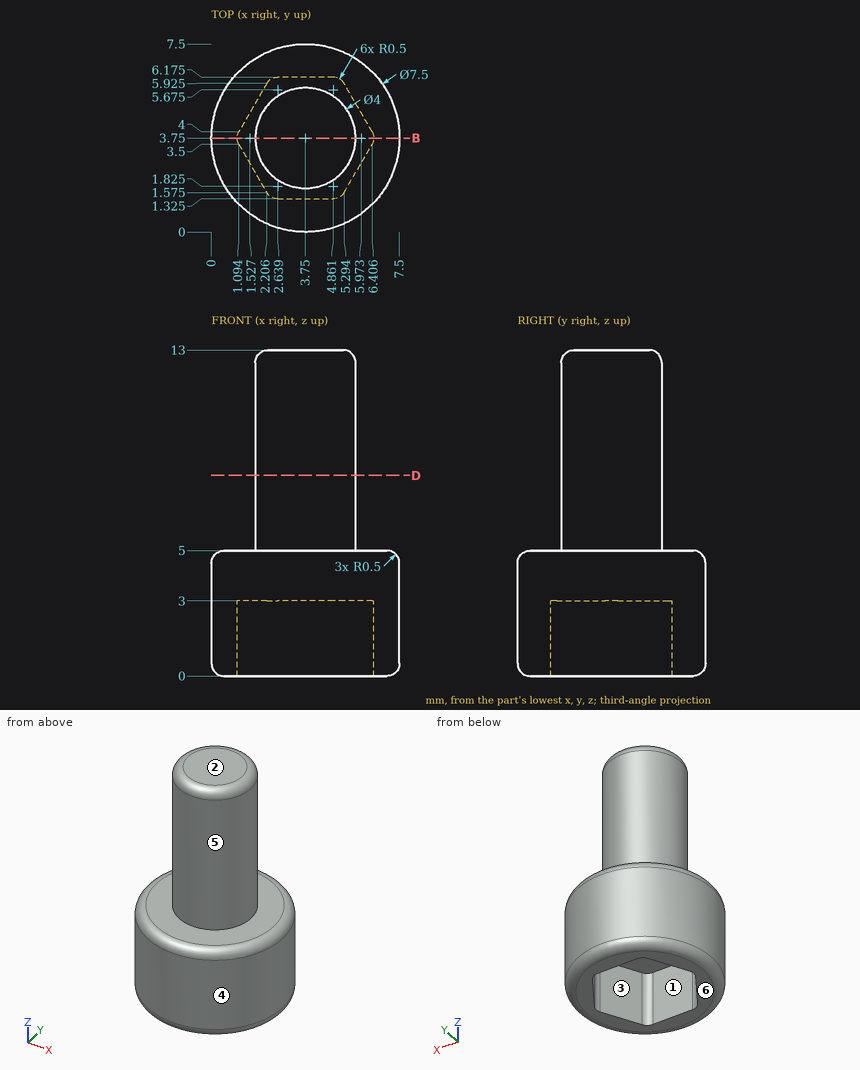
Part print with two shaded views. Sizes in mm from the minimum x, y, z corner. A direction names the side the tool comes from. Round coordinates to 2 decimals unless told otherwise and drop trailing zeros. Order: outer loops, then holes, each group sorted by start corner. A loop starts at its lowest first (then second) coordinate and runs counter-clockwise, first axis right, second up. Notation, with made-up numbers: (89.25, 70) - (108.25, 70) arc R21 ccw to (108.25, 85) - close; hole circle Ø8 at (-7.75, 78.25). An arc over 180 degrees is marked (long way). Answer as CSV lines item,"result". Start each with the question number.
1. Tool access for the marked faces 5 and 6: list every direction of +Z, -Z, +X, -X, +Y, -Y with a clear straight run to the whole face (end or side of a thin tool).
2. Saw through at D-D, the plane z = 8. Write the cut outline in (x, y), and give its area (3 significant figures).
3. Pull direction X, two halves, no side cores. Call the marked faces 1, 2, 3 and 4: +X half, -X half, draft (parallel to the pull), parting line (faces both ways), or undercut.
4. Drill centre lines: L1, parallel to Y at x = 3.75, z = 5.75; L2, parallel to Z at x = 3.5, y = 2.25; L3, parallel to Y at x = 5.5, z = 1.5 (1 decimal). Where is each one in solid material? Low to high. Write a range as [from, to].
5. Pin check, flat tip, straight feed: pin 1 (4 mm diameter, centred on x = 1, y = 6, fed in from +Z). Stop position of the tip, or through.
6. Saw through at B-B, the plane y = 3.75. Write the cut outline in (x, z).
Model answer:
1,face 5,"+Z"
1,face 6,"-Z, +X, -X, +Y, -Y"
2,outline,"circle Ø4 at (3.75, 3.75)"
2,area,"12.6 mm²"
3,face 1,"undercut"
3,face 2,"draft"
3,face 3,"undercut"
3,face 4,"parting line"
4,L1,"y = [1.75, 5.75]"
4,L2,"z = [3, 13]"
4,L3,"y = [0.4, 1.9], [5.6, 7.1]"
5,pin 1,"stops at z = 13"
6,outline,"(0, 0.5) arc R0.5 ccw to (0.5, 0) - (1.03, 0) - (1.03, 3) - (6.47, 3) - (6.47, 0) - (7, 0) arc R0.5 ccw to (7.5, 0.5) - (7.5, 4.5) arc R0.5 ccw to (7, 5) - (5.75, 5) - (5.75, 12.5) arc R0.5 ccw to (5.25, 13) - (2.25, 13) arc R0.5 ccw to (1.75, 12.5) - (1.75, 5) - (0.5, 5) arc R0.5 ccw to (0, 4.5) - close"
